from build123d import *

# Parameters (mm, degrees)
SKETCH1_R                       = 90
SKETCH1_R_2                     = 87
BOSS_EXTRUDE1_DEPTH             = 30
BOSS_EXTRUDE2_REACH             = 205.47
SKETCH2_W                       = 130
SKETCH2_H                       = 30
BOSS_EXTRUDE2_DIRECTION_2_DEPTH = 5
BOSS_EXTRUDE3_DEPTH             = 40


with BuildPart() as part:
    # Sketch1 → Boss-Extrude1 (new body)
    with BuildSketch(Plane.XY):
        Circle(SKETCH1_R)
        Circle(SKETCH1_R_2, mode=Mode.SUBTRACT)
    extrude(amount=BOSS_EXTRUDE1_DEPTH)

    # Boss-Extrude2: up to this face of the body
    boss_extrude2_end = part.part.faces().sort_by_distance((-90, 0, 15))[0]
    # Sketch2 → Boss-Extrude2 (add, up to the picked face)
    with BuildSketch(Plane(origin=(0, 90, 0), x_dir=(1, 0, 0), z_dir=(0, 1, 0)), mode=Mode.PRIVATE) as boss_extrude2_sk1:
        with Locations((0, -15)):
            Rectangle(SKETCH2_W, SKETCH2_H)
    boss_extrude2_tool1 = split(extrude(boss_extrude2_sk1.sketch, amount=-BOSS_EXTRUDE2_REACH, mode=Mode.PRIVATE), bisect_by=boss_extrude2_end, keep=Keep.BOTH, mode=Mode.PRIVATE)
    add(boss_extrude2_tool1.solids().sort_by(Axis((0, 90, 15), (0, -1, 0)))[0])
    add(boss_extrude2_tool1.solids().sort_by(Axis((0, 90, 15), (0, -1, 0)))[1])

    # Sketch2 → Boss-Extrude2 direction 2 (add)
    with BuildSketch(Plane(origin=(0, 90, 0), x_dir=(1, 0, 0), z_dir=(0, 1, 0))):
        with Locations((0, -15)):
            Rectangle(SKETCH2_W, SKETCH2_H)
    extrude(amount=BOSS_EXTRUDE2_DIRECTION_2_DEPTH)

    # Sketch3 → Boss-Extrude3 (add)
    with BuildSketch(Plane.XY.offset(30)):
        with BuildLine():
            Line((65, 95), (-65, 95))
            Line((-65, 95), (-65, 62.24949799))
            Line((-65, 62.24949799), (-65, 57.827329179))
            ThreePointArc((-65, 57.827329179), (0, 87), (65, 57.827329179))
            Line((65, 57.827329179), (65, 62.24949799))
            Line((65, 62.24949799), (65, 95))
        make_face()
    extrude(amount=BOSS_EXTRUDE3_DEPTH)

    # Mirror2: part across plane


with BuildPart() as part_1:
    add(part.part)
    add(part.part.mirror(Plane.XY.offset(70)))


solid = part_1.part
For this review, take the finished solid that the model builds, in its own axes (mm). Coordinates: 2 decimals unless noted, no trailing zeros. Loops run counter-clockwise (first coordinate to the right, second up) from the corner with the lowest first, then second, coordinate; pieces in that order, holes last. Notation, with made-up numbers: (50.25, -6.5) - (54.25, -6.5) arc R19 ccw to (54.25, 15.5) - close; hole circle Ø7 at (-10.75, -2.5). An arc over 180 degrees is marked (long way). Use a Markdown table: item, result. Add a question column.
Item 1: We need section D-D (z = 131.5). Give the boundary of the cut face in (x, y), and give its area (3 significant figures).
Item 2: For line 1 (X direction, y = 0, z = 7); line 2 (Y direction, x = 47, z = 123.5); line 3 (Y direction, x = 52, z = 24), list the stretches that pass through material, from the lowest coordinate up.
Item 3: We need section B-B (x = 0). Give the boundary of the cut face in (y, z), and give its area (3 significant figures).
Item 4: Mouldability with a two-part tool opening along Z and no side actions: class faces 1 (the face through (-2.94, -89.95, 125.21)), 2 (the face through (-7, -88, 30)), 3 (the face through (-27, 84, 140)), 4 (the face through (-7, -88, 110)) as pulls with the +Z half, pulls with the -Z half, needs draft (parallel to the pull), parting line crosses it, or undercut.
Item 5: We need section C-C (y = 68). Give the boundary of the cut face in (x, z).
Item 6: We need section A-A (y = 0). Give the boundary of the cut face in (x, z).
Item 7: Insertion check: pin 1 Ø6 at (y, z) = (-19.5, 117.5) entering from +X; pin 2 Ø18.5 at (y, z) = (70, 65.5) entering from -X; pin 3 Ø12 at (y, z) = (35.5, 125.5) entering from +X. Each pin has a flat end and moves straight along its axis. Give the tip position at first contact, or say it passes through.
Results list:
| question | item | result |
|---|---|---|
| 1 | outline | (-65, 62.25) arc R90 ccw (long way) to (65, 62.25) - (65, 95) - (-65, 95) - close; hole circle Ø174 at (0, 0) |
| 1 | area | 3,440 mm^2 |
| 2 | line 1 | x = -90 to -87, 87 to 90 |
| 2 | line 2 | y = -76.75 to -73.21, 73.21 to 95 |
| 2 | line 3 | y = -73.46 to -69.75, 69.75 to 95 |
| 3 | outline | (-90, 0) - (-87, 0) - (-87, 30) - (-90, 30) - close; (-90, 110) - (-87, 110) - (-87, 140) - (-90, 140) - close; (87, 0) - (95, 0) - (95, 140) - (87, 140) - close |
| 3 | area | 1,300 mm^2 |
| 4 | face 1 | needs draft |
| 4 | face 2 | undercut |
| 4 | face 3 | pulls with the +Z half |
| 4 | face 4 | undercut |
| 5 | outline | (-65, 0) - (-54.27, 0) - (-54.27, 140) - (-65, 140) - close; (54.27, 0) - (65, 0) - (65, 140) - (54.27, 140) - close |
| 6 | outline | (-90, 0) - (-87, 0) - (-87, 30) - (-90, 30) - close; (-90, 110) - (-87, 110) - (-87, 140) - (-90, 140) - close; (87, 0) - (90, 0) - (90, 30) - (87, 30) - close; (87, 110) - (90, 110) - (90, 140) - (87, 140) - close |
| 7 | pin 1 | stops at x = 88.47 |
| 7 | pin 2 | stops at x = -65 |
| 7 | pin 3 | stops at x = 85.03 |
